```python
from build123d import *

# Parameters (mm, degrees)
SKETCH1_R           = 2.032
BOSS_EXTRUDE1_DEPTH = 7.14375
SKETCH2_R           = 2.032
CUT_EXTRUDE1_DEPTH  = 22.135224042
FILLET1_R           = 0.396875


with BuildPart() as part:
    # Sketch1 → Boss-Extrude1 (new, symmetric)
    with BuildSketch(Plane(origin=(0, 0, 0), x_dir=(0, 0, -1), z_dir=(1, 0, 0))):
        with BuildLine():
            Line((-4.7625, 0), (-4.7625, 12.7))
            ThreePointArc((-4.7625, 12.7), (0, 17.4625), (4.7625, 12.7))
            Line((4.7625, 12.7), (4.7625, 0))
            ThreePointArc((4.7625, 0), (0, -4.7625), (-4.7625, 0))
        make_face()
        with Locations((0, 12.7)):
            Circle(SKETCH1_R, mode=Mode.SUBTRACT)
        Circle(SKETCH1_R, mode=Mode.SUBTRACT)
    extrude(amount=BOSS_EXTRUDE1_DEPTH, both=True)

    # Sketch2 → Cut-Extrude1 (cut, through all)
    with BuildSketch(Plane.XY.offset(4.7625)):
        with Locations((0, 6.35)):
            Circle(SKETCH2_R)
    extrude(amount=-CUT_EXTRUDE1_DEPTH, mode=Mode.SUBTRACT)

    # Fillet1
    fillet1_edges = [part.edges().sort_by_distance(p)[0] for p in [
        (7.14375, 17.4625, 0),
        (7.14375, 6.35, 4.7625),
        (7.14375, -4.7625, 0),
        (-7.14375, 6.35, 4.7625),
        (-7.14375, 17.4625, 0),
        (-7.14375, 6.35, -4.7625),
        (-7.14375, -4.7625, 0),
        (7.14375, 6.35, -4.7625),
    ]]
    fillet(fillet1_edges, radius=FILLET1_R)


solid = part.part
```
Part model, mm, in its own coordinate system. Round coordinates to 2 decimals unless told otherwise and drop trailing zeros. Loops run counter-clockwise (first coordinate to the right, second up) from the corner with the lowest first, then second, coordinate; pieces in that order, holes last.
Item 1: Cut at A-A, the plane x = 0. Give the cut face in (y, z) (1 decimal), then the cut area to 3 significant figures.
Item 2: Drill centre lines: line 1 (Y direction, x = 2.75, z = 0); line 2 (Z direction, x = -0.5, y = 12.75); line 3 (Y direction, x = 3.75, z = 1). Where is each one in solid material? Low to high.
Item 3: Cut at C-C, the plane y = 6.35. Give the cut face in (x, z).
Item 4: Mould opens along Y. For faces 1 (the face through (-0.1, 10.716, 0.44)), 2 (the face through (-7.144, 7, 0)), 3 (the face through (0.09, -4.76, -0.1)), 4 (the face through (0.09, 17.46, 0.1)) say: +Y half, -Y half, draft (parallel to the pull), parting line (faces both ways), or undercut.
Item 5: Cut at D-D, the plane x = 4. Give the cut face in (y, z) (1 decimal), then the cut area to 3 significant figures.
Item 6: Cut at B-B, the plane z = 0. Give the cut face in (x, y), then the cut area to 3 significant figures.
Item 7: Drop flat-ended pins along their axis: P1, Ø1.5, axis at x = 4.5, y = 13.5, coming from the +Z side; P2, Ø1.5, axis at x = 2.5, z = -2.5, coming from the -Y side; P3, Ø1.5, axis at x = -0.5, z = -3, coming from the -Y side. Give the stop position or say it passes through.
A:
1. outline: (0, -4.8) - (4.3, -4.8) - (4.3, 4.8) - (0, 4.8) arc R4.8 ccw to start; (8.4, -4.8) - (12.7, -4.8) arc R4.8 ccw to (12.7, 4.8) - (8.4, 4.8) - close; hole circle Ø4.1 at (0, 0); hole circle Ø4.1 at (12.7, 0)
1. area: 128 mm2
2. line 1: y = -4.76 to -2.03, 2.03 to 10.67, 14.73 to 17.46
2. line 2: z = -4.76 to -2.03, 2.03 to 4.76
2. line 3: y = -4.66 to -1.77, 1.77 to 10.93, 14.47 to 17.36
3. outline: (-7.14, -4.37) arc R0.4 ccw to (-6.75, -4.76) - (-2.03, -4.76) - (-2.03, 4.76) - (-6.75, 4.76) arc R0.4 ccw to (-7.14, 4.37) - close; (2.03, -4.76) - (6.75, -4.76) arc R0.4 ccw to (7.14, -4.37) - (7.14, 4.37) arc R0.4 ccw to (6.75, 4.76) - (2.03, 4.76) - close
4. face 1: undercut
4. face 2: draft
4. face 3: -Y half
4. face 4: +Y half
5. outline: (0, -4.8) - (12.7, -4.8) arc R4.8 ccw to (12.7, 4.8) - (0, 4.8) arc R4.8 ccw to start; hole circle Ø4.1 at (0, 0); hole circle Ø4.1 at (12.7, 0)
5. area: 166 mm2
6. outline: (-7.14, -4.37) arc R0.4 ccw to (-6.75, -4.76) - (6.75, -4.76) arc R0.4 ccw to (7.14, -4.37) - (7.14, -2.03) - (-7.14, -2.03) - close; (-7.14, 2.03) - (7.14, 2.03) - (7.14, 10.67) - (-7.14, 10.67) - close; (-7.14, 14.73) - (7.14, 14.73) - (7.14, 17.07) arc R0.4 ccw to (6.75, 17.46) - (-6.75, 17.46) arc R0.4 ccw to (-7.14, 17.07) - close; hole circle Ø4.06 at (0, 6.35)
6. area: 188 mm2
7. P1: stops at z = 4.76
7. P2: stops at y = -4.43
7. P3: stops at y = -4.2
